Input: part model. Units: mm. Frame: model coordinates. A direction names the side the tool comes from. Coordinates: 2 decimals unless noted, no trailing zeros. Write each loop counter-clockwise with the first axis right and the second up, starting at its lowest first coordinate (ties: lowest second). Pieces come first, ordered by that corner, then holes. Notation, with made-up numbers: (-18.5, 76) - (6.5, 76) arc R29 cw to (6.5, 115) - close; hole circle Ø3 at (-39, 65.5). An arc over 180 degrees is marked (long way). Use CSV: the item, a comma, the result in double quotes.
```python
from build123d import *

# Parameters (mm, degrees)
F0_R     = 1.5
F1_DEPTH = 4
F2_DEPTH = 4
F3_R     = 0.65
F4_DEPTH = 3


with BuildPart() as f1:
    # F0 (on Front) → F1 (new body)
    with BuildSketch(Plane.XZ):
        Polygon((-7.5, -12.5), (7.5, -12.5), (7.5, 22.5), (2, 22.5), (2, 27.5), (-2, 27.5), (-2, 22.5), (-7.5, 22.5), align=None)
        with Locations((0, -5.542802)):
            Circle(F0_R, mode=Mode.SUBTRACT)
    extrude(amount=F1_DEPTH)

    # F0 (on Front) → F2 (join)
    with BuildSketch(Plane.XZ):
        Polygon((-7.5, -12.5), (7.5, -12.5), (7.5, 22.5), (2, 22.5), (2, 27.5), (-2, 27.5), (-2, 22.5), (-7.5, 22.5), align=None)
        with Locations((0, -5.542802)):
            Circle(F0_R, mode=Mode.SUBTRACT)
    extrude(amount=F2_DEPTH)

    # F3 (on face) → F4 (cut)
    with BuildSketch(Plane.XY.offset(27.5)):
        with Locations((0, -2)):
            Circle(F3_R)
    extrude(amount=-F4_DEPTH, mode=Mode.SUBTRACT)


solid = f1.part
```
(1) Ray query, probe 1 along Y at (x, z) = (0, 26.5); probe 2 along Z at (x, y) = (0, -1.2); probe 3 along Z at (x, y) = (0, -1.7). Return the intervals inside material, ascending. Write a range as from..to.
Check values:
probe 1,"-4..-2.65, -1.35..0"
probe 2,"-12.5..-7.04, -4.04..27.5"
probe 3,"-12.5..-7.04, -4.04..24.5"
(2) Cut plane C-C on y = -2. Return loops of the section in (x, z), and give its area (3 significant figures).
Check values:
outline,"(-7.5, -12.5) - (7.5, -12.5) - (7.5, 22.5) - (2, 22.5) - (2, 27.5) - (0.65, 27.5) - (0.65, 24.5) - (-0.65, 24.5) - (-0.65, 27.5) - (-2, 27.5) - (-2, 22.5) - (-7.5, 22.5) - close; hole circle Ø3 at (0, -5.54)"
area,"534 mm^2"
(3) Cut plane B-B on z = 25. Return loops of the section in (x, y), and give its area (3 significant figures).
Check values:
outline,"(-2, -4) - (2, -4) - (2, 0) - (-2, 0) - close; hole circle Ø1.3 at (0, -2)"
area,"14.7 mm^2"
(4) Draft query along X for faces 1 (the flat face through (2, -2, 25)), 2 (the flat face through (0, -2, -12.5)), 3 (the flat face through (0, -2, 24.5)). Return one class per face: pulls with the +X half, pulls with the -X half, needs draft (parallel to the pull), parting line crosses it, or undercut.
Check values:
face 1,"pulls with the +X half"
face 2,"needs draft"
face 3,"undercut"
(5) Cut plane A-A on x = 0. Return loops of the section in (y, z).
Check values:
outline,"(-4, -12.5) - (0, -12.5) - (0, -7.04) - (-4, -7.04) - close; (-4, -4.04) - (0, -4.04) - (0, 27.5) - (-1.35, 27.5) - (-1.35, 24.5) - (-2.65, 24.5) - (-2.65, 27.5) - (-4, 27.5) - close"
(6) Cut plane D-D on x = 4.25. Return loops of the section in (y, z).
Check values:
outline,"(-4, -12.5) - (0, -12.5) - (0, 22.5) - (-4, 22.5) - close"
(7) Pin query (flat end, axial travel): pin 1 Ø1.2 at (x, y) = (5.5, -2.5) entering from +Z; pin 2 Ø2.5 at (x, z) = (0, -5.54) entering from +Y; pin 3 Ø2 at (y, z) = (-1, 24) entering from -X; pin 4 Ø2 at (y, z) = (-2, 26) entering from +X. Return the tip coordinate at first contact, or that it passes through.
Check values:
pin 1,"z = 22.5"
pin 2,"through"
pin 3,"x = -2"
pin 4,"x = 2"
(8) Reachability of faces 4 (the flat face through (0, 0, 8)), 5 (the flat face through (1, -2, 27.5)), 6 (the flat face through (-5, -2, 22.5)), 7 (the cylindrical face through (-0.141, -2.635, 26.021)), 8 (the flat face through (5, -2, 22.5)) from +Z, -Z, +X, -X, +Y, -Y: full face, straight path, thin tool, end or side. Return the list, or none.
Check values:
face 4,"+Z, -Z, +X, -X, +Y"
face 5,"+Z, +X, -X, +Y, -Y"
face 6,"+Z, -X, +Y, -Y"
face 7,"+Z"
face 8,"+Z, +X, +Y, -Y"
